Work out the finished part from the listing and answer in its coordinate system (mm). Face numbers are marked on the shaded views. A direction names the side the tool comes from. Give positions to 0.01 mm unless a question says otherwise; leave off trailing zeros. Write each loop counter-clockwise with the first axis right and the second up, starting at its lowest first coordinate (ties: lowest second). Pieces come first, ordered by that corner, then holes. Notation, with made-up numbers: (31, 73.25) -> (49, 73.25) arc R20 cw to (49, 88.25) -> close; hole circle Ø7 at (68, -32). An arc over 180 degrees is marked (long way). Write item = value, one per line. Start each with the question number.
from build123d import *

# Parameters (mm, degrees)
F0_R     = 46.99
F1_DEPTH = 1.397
F3_DEPTH = 25.4
F4_R     = 6.35
F5_DEPTH = 7.62
F6_SIZE  = 0.508
F8_DEPTH = 20.32


with BuildPart() as f1:
    # F0 (on Top) → F1 (new body)
    with BuildSketch(Plane.XY):
        Circle(F0_R)
    extrude(amount=F1_DEPTH)

    # F2 (on face) → F3 (cut)
    with BuildSketch(Plane(origin=(0, 0, 0), x_dir=(1, 0, 0), z_dir=(0, 0, -1))):
        Polygon((2.4929984624, 4.318), (-2.4929984624, 4.318), (-4.9859969247, 0), (-2.4929984624, -4.318), (2.4929984624, -4.318), (4.9859969247, 0), align=None)
    extrude(amount=-F3_DEPTH, mode=Mode.SUBTRACT)

    # F4 (on face) → F5 (join)
    with BuildSketch(Plane.XY.offset(1.397)):
        Circle(F4_R)
        Polygon((2.4929984624, 4.318), (4.9859969247, 0), (2.4929984624, -4.318), (-2.4929984624, -4.318), (-4.9859969247, 0), (-2.4929984624, 4.318), align=None, mode=Mode.SUBTRACT)
    extrude(amount=F5_DEPTH)

    # F6
    f6_edges = [f1.edges().sort_by_distance(p)[0] for p in [
        (-6.35, 0, 9.017),
    ]]
    chamfer(f6_edges, length=F6_SIZE)

    # F7 (on face) → F8 (join)
    with BuildSketch(Plane.XY.offset(1.397)):
        with BuildLine():
            ThreePointArc((25.4, 0), (35.2612826312, 9.5139210825), (41.7364588819, 21.59))
            ThreePointArc((41.7364588819, 21.59), (40.9458823261, 23.0541714346), (40.1039614528, 24.4894339623))
            ThreePointArc((40.1039614528, 24.4894339623), (34.7338091215, 11.6119097242), (25.3682301314, 1.27))
            Line((25.3682301314, 1.27), (25.4, 0))
        make_face()
        with BuildLine():
            ThreePointArc((21.9970452561, 12.7), (25.7802059874, 25.8699386627), (25.3498336557, 39.5657179087))
            ThreePointArc((25.3498336557, 39.5657179087), (23.9330885575, 40.4384392886), (22.4863324294, 41.260452662))
            ThreePointArc((22.4863324294, 41.260452662), (24.2744062074, 27.4231133684), (21.3345317428, 13.7839673285))
            Line((21.3345317428, 13.7839673285), (21.9970452561, 12.7))
        make_face()
        with BuildLine():
            ThreePointArc((12.7, 21.9970452561), (9.3913439685, 35.2941270699), (2.1707409732, 46.9398336557))
            ThreePointArc((2.1707409732, 46.9398336557), (0.5074430375, 46.9872599921), (-1.1564912092, 46.9757663917))
            ThreePointArc((-1.1564912092, 46.9757663917), (7.3106957532, 35.8863159315), (11.5842628029, 22.6045317428))
            Line((11.5842628029, 22.6045317428), (12.7, 21.9970452561))
        make_face()
        with BuildLine():
            ThreePointArc((0, 25.4), (-9.5139210825, 35.2612826312), (-21.59, 41.7364588819))
            ThreePointArc((-21.59, 41.7364588819), (-23.0541714346, 40.9458823261), (-24.4894339623, 40.1039614528))
            ThreePointArc((-24.4894339623, 40.1039614528), (-11.6119097242, 34.7338091215), (-1.27, 25.3682301314))
            Line((-1.27, 25.3682301314), (0, 25.4))
        make_face()
        with BuildLine():
            ThreePointArc((-12.7, 21.9970452561), (-25.8699386627, 25.7802059874), (-39.5657179087, 25.3498336557))
            ThreePointArc((-39.5657179087, 25.3498336557), (-40.4384392886, 23.9330885575), (-41.260452662, 22.4863324294))
            ThreePointArc((-41.260452662, 22.4863324294), (-27.4231133684, 24.2744062074), (-13.7839673285, 21.3345317428))
            Line((-13.7839673285, 21.3345317428), (-12.7, 21.9970452561))
        make_face()
        with BuildLine():
            ThreePointArc((-21.9970452561, 12.7), (-35.2941270699, 9.3913439685), (-46.9398336557, 2.1707409732))
            ThreePointArc((-46.9398336557, 2.1707409732), (-46.9872599921, 0.5074430375), (-46.9757663917, -1.1564912092))
            ThreePointArc((-46.9757663917, -1.1564912092), (-35.8863159315, 7.3106957532), (-22.6045317428, 11.5842628029))
            Line((-22.6045317428, 11.5842628029), (-21.9970452561, 12.7))
        make_face()
        with BuildLine():
            ThreePointArc((-41.7364588819, -21.59), (-40.9458823261, -23.0541714346), (-40.1039614528, -24.4894339623))
            ThreePointArc((-40.1039614528, -24.4894339623), (-34.7338091215, -11.6119097242), (-25.3682301314, -1.27))
            Line((-25.3682301314, -1.27), (-25.4, 0))
            ThreePointArc((-25.4, 0), (-35.2612826312, -9.5139210825), (-41.7364588819, -21.59))
        make_face()
        with BuildLine():
            ThreePointArc((-25.3498336557, -39.5657179087), (-23.9330885575, -40.4384392886), (-22.4863324294, -41.260452662))
            ThreePointArc((-22.4863324294, -41.260452662), (-24.2744062074, -27.4231133684), (-21.3345317428, -13.7839673285))
            Line((-21.3345317428, -13.7839673285), (-21.9970452561, -12.7))
            ThreePointArc((-21.9970452561, -12.7), (-25.7802059874, -25.8699386627), (-25.3498336557, -39.5657179087))
        make_face()
        with BuildLine():
            ThreePointArc((-2.1707409732, -46.9398336557), (-0.5074430375, -46.9872599921), (1.1564912092, -46.9757663917))
            ThreePointArc((1.1564912092, -46.9757663917), (-7.3106957532, -35.8863159315), (-11.5842628029, -22.6045317428))
            Line((-11.5842628029, -22.6045317428), (-12.7, -21.9970452561))
            ThreePointArc((-12.7, -21.9970452561), (-9.3913439685, -35.2941270699), (-2.1707409732, -46.9398336557))
        make_face()
        with BuildLine():
            ThreePointArc((21.59, -41.7364588819), (23.0541714346, -40.9458823261), (24.4894339623, -40.1039614528))
            ThreePointArc((24.4894339623, -40.1039614528), (11.6119097242, -34.7338091215), (1.27, -25.3682301314))
            Line((1.27, -25.3682301314), (0, -25.4))
            ThreePointArc((0, -25.4), (9.5139210825, -35.2612826312), (21.59, -41.7364588819))
        make_face()
        with BuildLine():
            ThreePointArc((39.5657179087, -25.3498336557), (40.4384392886, -23.9330885575), (41.260452662, -22.4863324294))
            ThreePointArc((41.260452662, -22.4863324294), (27.4231133684, -24.2744062074), (13.7839673285, -21.3345317428))
            Line((13.7839673285, -21.3345317428), (12.7, -21.9970452561))
            ThreePointArc((12.7, -21.9970452561), (25.8699386627, -25.7802059874), (39.5657179087, -25.3498336557))
        make_face()
        with BuildLine():
            ThreePointArc((46.99, 0), (46.9864414632, 0.5782893983), (46.9757663917, 1.1564912092))
            ThreePointArc((46.9757663917, 1.1564912092), (35.8863159315, -7.3106957532), (22.6045317428, -11.5842628029))
            Line((22.6045317428, -11.5842628029), (21.9970452561, -12.7))
            ThreePointArc((21.9970452561, -12.7), (35.2941270699, -9.3913439685), (46.9398336557, -2.1707409732))
            ThreePointArc((46.9398336557, -2.1707409732), (46.9774567398, -1.085660287), (46.99, 0))
        make_face()
    extrude(amount=F8_DEPTH)


solid = f1.part
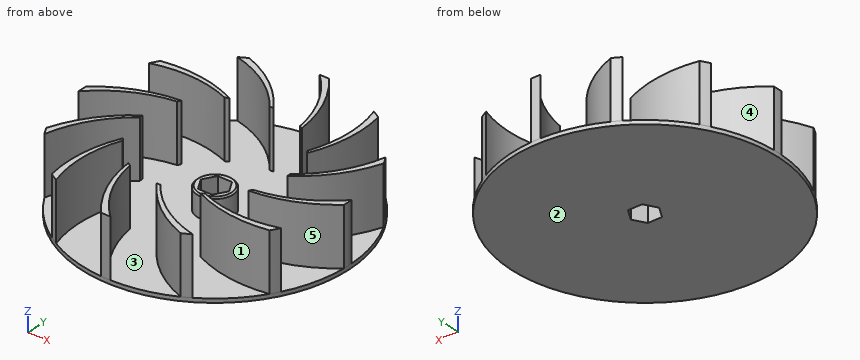
(1) A cutting plane is placed at D-D, the plane x = -35.5. Write down the section's boundary in (y, z) (3 decimals), then the cut area to 3 significant figures.
(2) A cutting plane is placed at B-B, the plane y = -18.5. Write down the section's boundary in (x, z).
(3) For the marked faces 1 and 2, determine the directions among +Z, -Z, +X, -X, +Y, -Y from which every point of the face is accessible in a straight line to the end or side of a thin tool.
(4) Determine the mould class of the marked faces 3, 4 and 5 for opening direction X: pulls with the +X half, pulls with the -X half, needs draft (parallel to the pull), parting line crosses it, or undercut.
(5) A cutting plane is placed at A-A, the plane z = 4. State how many separate pieces and enclosed holes the cut face has, then the cut area to 3 significant figures.
(6) Each of these flat-tipped pins is pushed along its axis until it touches: pin 1 (10 mm diameter, centred on y = 6.5, z = 16.5, fed in from -X); pin 2 (1 mm diameter, centred on y = -5.5, z = 10.5, fed in from -X); pin 3 (9.5 mm diameter, centred on x = -2.5, y = 0.5, fed in from +Z). Where does it stop, or does it pass through?
(7) Find the intervals of material crossed by line 1 along X through (y, z) = (-36.5, 10); line 2 along Y through (x, z) = (-37.5, 17); line 3 along X through (y, z) = (-32, 6), in increasing order.
Results list:
q1.outline = (-30.787, 0) -> (30.787, 0) -> (30.787, 1.397) -> (25.925, 1.397) -> (25.925, 21.717) -> (23.817, 21.717) -> (23.817, 1.397) -> (9.304, 1.397) -> (9.304, 21.717) -> (7.51, 21.717) -> (7.51, 1.397) -> (-9.832, 1.397) -> (-9.832, 21.717) -> (-12.868, 21.717) -> (-12.868, 1.397) -> (-30.787, 1.397) -> close
q1.area = 227 mm²
q2.outline = (-43.2, 0) -> (43.2, 0) -> (43.2, 1.4) -> (-22.91, 1.4) -> (-22.91, 21.72) -> (-24.21, 21.72) -> (-24.21, 1.4) -> (-38.24, 1.4) -> (-38.24, 21.72) -> (-40.52, 21.72) -> (-40.52, 1.4) -> (-43.2, 1.4) -> close
q3.face_1 = +Z
q3.face_2 = -Z, +X, -X, +Y, -Y
q4.face_3 = undercut
q4.face_4 = pulls with the -X half
q4.face_5 = pulls with the +X half
q5.separate_pieces = 13
q5.enclosed_holes = 1
q5.area = 614 mm²
q6.pin_1 = -46.97
q6.pin_2 = -32.3
q6.pin_3 = 9.02
q7.line_1 = -25.82 to -23.65, -8.86 to -6.98, 11.24 to 14.68
q7.line_2 = -16.74 to -12.76, 6.42 to 8.39, 23.45 to 25.69
q7.line_3 = -26.12 to -24.21, -10.63 to -9.09, 5.68 to 7.8
